Build history of the part. All positions in model axes, mm. A direction names the side the tool comes from. Coordinates: 2 decimals unless noted, no trailing zeros. Write each loop counter-clockwise with the first axis right and the second up, starting at its lowest first coordinate (ties: lowest second). Pieces come first, ordered by that corner, then holes.
```python
from build123d import *

# Parameters (mm, degrees)
F1_DEPTH = 7.8105
F0_R     = 9.37895
F2_DEPTH = 1.5494
F4_D     = 8.7249
F5_SIZE  = 1.27


# Not quite as in the source:
# - a fillet or chamfer that OpenCascade refuses, or shapes differently, is made with other operations: its cross-section is extruded or revolved along the edge and cut away or added


with BuildPart() as f1:
    # F0 (on Top) → F1 (new body)
    with BuildSketch(Plane.XY):
        Polygon((4.2291, 7.3250160703), (-4.2291, 7.3250160703), (-8.4582, 0), (-4.2291, -7.3250160703), (4.2291, -7.3250160703), (8.4582, 0), align=None)
    extrude(amount=F1_DEPTH)

    # F0 (on Top) → F2 (join)
    with BuildSketch(Plane.XY):
        Circle(F0_R)
        Polygon((-8.4582, 0), (-4.2291, 7.3250160703), (4.2291, 7.3250160703), (8.4582, 0), (4.2291, -7.3250160703), (-4.2291, -7.3250160703), align=None, mode=Mode.SUBTRACT)
    extrude(amount=F2_DEPTH)

    # F3: fillet of radius 1.016 on 1 edges, made by hand


with BuildPart() as f3_tool2:
    # F3_s3 → F3_t4 (revolve)
    with BuildSketch(Plane.XZ):
        with BuildLine():
            ThreePointArc((8.36295, 1.5494), (9.0813704897, 1.2518204897), (9.37895, 0.5334))
            Line((9.37895, 0.5334), (9.37895, 1.5494))
            Line((9.37895, 1.5494), (8.36295, 1.5494))
        make_face()
    revolve(axis=Axis((0, 0, 1.5494), (0, 0, 1)))

    split(bisect_by=Plane(origin=(6.34365, 3.6625080351, 0), x_dir=(0, 0, 1), z_dir=(0.8660254038, 0.5, 0)), keep=Keep.TOP)


with BuildPart() as f1_1:
    add(f1.part)

    # F3_t1: cut F3_tool2
    add(f3_tool2.part, mode=Mode.SUBTRACT)


with BuildPart() as f3_tool7:
    # F3_s8 → F3_t9 (revolve)
    with BuildSketch(Plane.XZ):
        with BuildLine():
            ThreePointArc((8.36295, 1.5494), (9.0813704897, 1.2518204897), (9.37895, 0.5334))
            Line((9.37895, 0.5334), (9.37895, 1.5494))
            Line((9.37895, 1.5494), (8.36295, 1.5494))
        make_face()
    revolve(axis=Axis((0, 0, 1.5494), (0, 0, 1)))

    split(bisect_by=Plane(origin=(6.34365, -3.6625080351, 0), x_dir=(0, 0, 1), z_dir=(0.8660254038, -0.5, 0)), keep=Keep.TOP)


with BuildPart() as f1_2:
    add(f1_1.part)

    # F3_t6: cut F3_tool7
    add(f3_tool7.part, mode=Mode.SUBTRACT)


with BuildPart() as f3_tool12:
    # F3_s13 → F3_t14 (revolve)
    with BuildSketch(Plane.XZ):
        with BuildLine():
            ThreePointArc((8.36295, 1.5494), (9.0813704897, 1.2518204897), (9.37895, 0.5334))
            Line((9.37895, 0.5334), (9.37895, 1.5494))
            Line((9.37895, 1.5494), (8.36295, 1.5494))
        make_face()
    revolve(axis=Axis((0, 0, 1.5494), (0, 0, 1)))

    split(bisect_by=Plane.XZ.offset(-7.3250160703), keep=Keep.BOTTOM)


with BuildPart() as f1_3:
    add(f1_2.part)

    # F3_t11: cut F3_tool12
    add(f3_tool12.part, mode=Mode.SUBTRACT)


with BuildPart() as f3_tool17:
    # F3_s18 → F3_t19 (revolve)
    with BuildSketch(Plane.XZ):
        with BuildLine():
            ThreePointArc((8.36295, 1.5494), (9.0813704897, 1.2518204897), (9.37895, 0.5334))
            Line((9.37895, 0.5334), (9.37895, 1.5494))
            Line((9.37895, 1.5494), (8.36295, 1.5494))
        make_face()
    revolve(axis=Axis((0, 0, 1.5494), (0, 0, 1)))

    split(bisect_by=Plane.XZ.offset(7.3250160703), keep=Keep.TOP)


with BuildPart() as f1_4:
    add(f1_3.part)

    # F3_t16: cut F3_tool17
    add(f3_tool17.part, mode=Mode.SUBTRACT)


with BuildPart() as f3_tool22:
    # F3_s23 → F3_t24 (revolve)
    with BuildSketch(Plane.XZ):
        with BuildLine():
            ThreePointArc((8.36295, 1.5494), (9.0813704897, 1.2518204897), (9.37895, 0.5334))
            Line((9.37895, 0.5334), (9.37895, 1.5494))
            Line((9.37895, 1.5494), (8.36295, 1.5494))
        make_face()
    revolve(axis=Axis((0, 0, 1.5494), (0, 0, 1)))

    split(bisect_by=Plane(origin=(-6.34365, 3.6625080351, 0), x_dir=(0, 0, 1), z_dir=(-0.8660254038, 0.5, 0)), keep=Keep.TOP)


with BuildPart() as f1_5:
    add(f1_4.part)

    # F3_t21: cut F3_tool22
    add(f3_tool22.part, mode=Mode.SUBTRACT)


with BuildPart() as f3_tool27:
    # F3_s28 → F3_t29 (revolve)
    with BuildSketch(Plane.XZ):
        with BuildLine():
            ThreePointArc((8.36295, 1.5494), (9.0813704897, 1.2518204897), (9.37895, 0.5334))
            Line((9.37895, 0.5334), (9.37895, 1.5494))
            Line((9.37895, 1.5494), (8.36295, 1.5494))
        make_face()
    revolve(axis=Axis((0, 0, 1.5494), (0, 0, 1)))

    split(bisect_by=Plane(origin=(-6.34365, -3.6625080351, 0), x_dir=(0, 0, 1), z_dir=(-0.8660254038, -0.5, 0)), keep=Keep.TOP)


with BuildPart() as f1_6:
    add(f1_5.part)

    # F3_t26: cut F3_tool27
    add(f3_tool27.part, mode=Mode.SUBTRACT)

    # F4 (through all)
    with Locations(Plane(origin=(0, 0, 0), x_dir=(1, 0, 0), z_dir=(0, 0, -1))):
        with Locations((0, 0)):
            Hole(F4_D / 2)

    # F5
    f5_edges = [f1_6.edges().sort_by_distance(p)[0] for p in [
        (0, 7.325016, 7.8105),
        (6.34365, 3.662508, 7.8105),
        (6.34365, -3.662508, 7.8105),
        (0, -7.325016, 7.8105),
        (-6.34365, -3.662508, 7.8105),
        (-6.34365, 3.662508, 7.8105),
        (-4.36245, 0, 7.8105),
        (-4.36245, 0, 0),
    ]]
    chamfer(f5_edges, length=F5_SIZE)


solid = f1_6.part
```
1. Saw through at B-B on z = 3.25. List the corners of the cut face in (x, y), plus the area to 3 significant figures.
Computed values:
outline: (-8.46, 0) - (-4.23, -7.33) - (4.23, -7.33) - (8.46, 0) - (4.23, 7.33) - (-4.23, 7.33) - close; hole circle Ø8.72 at (0, 0)
area: 126 mm2
2. Mould opens along X. For faces 6 (the face through (3.462, 2.654, 3.942)), 7 (the face through (7, 4, 1.549)), 8 (the face through (5.77, -3.4, 7.17)) say: +X half, -X half, draft (parallel to the pull), parting line (faces both ways), or undercut.
Computed values:
face 6: undercut
face 7: draft
face 8: +X half
3. Probe line 1 along Y through (x, z) = (0, 3.4); line 2 along Z through (x, y) = (-8.5, -0.25); line 3 along Y through (x, z) = (-1, 0.5). List the from-to ranges inside material, lowest first.
Computed values:
line 1: y = -7.33 to -4.36, 4.36 to 7.33
line 2: z = 0 to 1.54
line 3: y = -9.33 to -5.03, 5.03 to 9.33
4. 3-axis set-ups, long thin cutter, end or side, ignore diameter. For faces 1 (the face through (-7, -4, 1.549)), 2 (the face through (0, -7.325, 4)), 3 (the face through (7, -4, 1.549)), 4 (the face through (-7, 4, 1.549)), 5 (the face through (0, 7.325, 4)): which of +Z, -Z, +X, -X, +Y, -Y reach the whole face in a straight line?
Computed values:
face 1: +Z, -X, -Y
face 2: +Z, +X, -X, -Y
face 3: +Z, +X, -Y
face 4: +Z, -X, +Y
face 5: +Z, +X, -X, +Y
5. Flat gauge pins, fed straight in: pin 1 (2 mm diameter, centred on x = -6.5, y = 3.5, fed in from +Z); pin 2 (3 mm diameter, centred on x = 7, y = 4, fed in from +Z); pin 3 (4 mm diameter, centred on x = 0, z = 4.5, fed in from -Y) (3 decimals). Where does each tip first touch, or does it go through?
Computed values:
pin 1: stops at z = 7.49
pin 2: stops at z = 7.3
pin 3: stops at y = -7.325
6. Saw through at A-A on x = 0. List the corners of the cut face in (y, z), plus the area to 3 significant figures.
Computed values:
outline: (-9.38, 0) - (-5.63, 0) - (-4.36, 1.27) - (-4.36, 6.54) - (-5.63, 7.81) - (-6.06, 7.81) - (-7.33, 6.54) - (-7.33, 1.55) - (-8.36, 1.55) arc R1.02 ccw to (-9.38, 0.53) - close; (4.36, 1.27) - (5.63, 0) - (9.38, 0) - (9.38, 0.53) arc R1.02 ccw to (8.36, 1.55) - (7.33, 1.55) - (7.33, 6.54) - (6.06, 7.81) - (5.63, 7.81) - (4.36, 6.54) - close
area: 47.4 mm2
